The listing builds one solid part. Answer for the finished solid, in the listing's coordinates (mm). Face numbers are marked on the shaded views. A direction names the side the tool comes from. Round coordinates to 2 decimals unless told otherwise and drop trailing zeros. Write each loop counter-clockwise with the first axis right and the second up, starting at its lowest first coordinate (ties: lowest second). Pieces come first, ordered by that corner, then holes. Notation, with made-up numbers: (78, 7.25) - (97, 7.25) arc R17 ccw to (97, 28.25) - close; hole circle Ø4 at (-35.75, -33.75). An arc over 180 degrees is marked (long way). Return JSON: item names as keys, results as strings. Group by question number.
from build123d import *

# Parameters (mm, degrees)
BOSS_EXTRUDE1_DEPTH     = 110
BOSS_EXTRUDE2_START     = -105.9
BOSS_EXTRUDE2_DEPTH     = 211.8
CUT_EXTRUDE1_REACH      = 226.526
SKETCH3_R               = 3.175
F_1_4_CLEARANCE_HOLE1_D = 6.7564


with BuildPart() as part:
    # Sketch1 → Boss-Extrude1 (new body)
    with BuildSketch(Plane(origin=(0, 0, 0), x_dir=(1, 0, 0), z_dir=(0, 1, 0))):
        with BuildLine():
            Line((-14.05, 19.05), (14.05, 19.05))
            ThreePointArc((14.05, 19.05), (17.585533906, 17.585533906), (19.05, 14.05))
            Line((19.05, 14.05), (19.05, -14.05))
            ThreePointArc((19.05, -14.05), (17.585533906, -17.585533906), (14.05, -19.05))
            Line((14.05, -19.05), (-14.05, -19.05))
            ThreePointArc((-14.05, -19.05), (-17.585533906, -17.585533906), (-19.05, -14.05))
            Line((-19.05, -14.05), (-19.05, 14.05))
            ThreePointArc((-19.05, 14.05), (-17.585533906, 17.585533906), (-14.05, 19.05))
        make_face()
        with BuildLine():
            Line((-15.875, 14.05), (-15.875, -14.05))
            ThreePointArc((-15.875, -14.05), (-15.340469876, -15.340469876), (-14.05, -15.875))
            Line((-14.05, -15.875), (14.05, -15.875))
            ThreePointArc((14.05, -15.875), (15.340469876, -15.340469876), (15.875, -14.05))
            Line((15.875, -14.05), (15.875, 14.05))
            ThreePointArc((15.875, 14.05), (15.340469876, 15.340469876), (14.05, 15.875))
            Line((14.05, 15.875), (-14.05, 15.875))
            ThreePointArc((-14.05, 15.875), (-15.340469876, 15.340469876), (-15.875, 14.05))
        make_face(mode=Mode.SUBTRACT)
    extrude(amount=BOSS_EXTRUDE1_DEPTH)


with BuildPart() as body_2:
    # Mirror2: mirrored copy
    add(part.part.mirror(Plane(origin=(86.85, 0, 0), x_dir=(0, 0, 1), z_dir=(1, 0, 0))))


with BuildPart() as part_1:
    add(part.part)

    add(body_2.part)  # Boss-Extrude2 merges body 2
    # Sketch2 → Boss-Extrude2 (add)
    with BuildSketch(Plane(origin=(86.85, 0, 0), x_dir=(0, 0, -1), z_dir=(1, 0, 0)).offset(BOSS_EXTRUDE2_START)):
        with BuildLine():
            Line((-29.05, 148.1), (-0.95, 148.1))
            ThreePointArc((-0.95, 148.1), (2.585533906, 146.635533906), (4.05, 143.1))
            Line((4.05, 143.1), (4.05, 115))
            ThreePointArc((4.05, 115), (2.585533906, 111.464466094), (-0.95, 110))
            Line((-0.95, 110), (-29.05, 110))
            ThreePointArc((-29.05, 110), (-32.585533906, 111.464466094), (-34.05, 115))
            Line((-34.05, 115), (-34.05, 143.1))
            ThreePointArc((-34.05, 143.1), (-32.585533906, 146.635533906), (-29.05, 148.1))
        make_face()
        with BuildLine():
            Line((-30.875, 143.1), (-30.875, 115))
            ThreePointArc((-30.875, 115), (-30.340469876, 113.709530124), (-29.05, 113.175))
            Line((-29.05, 113.175), (-0.95, 113.175))
            ThreePointArc((-0.95, 113.175), (0.340469876, 113.709530124), (0.875, 115))
            Line((0.875, 115), (0.875, 143.1))
            ThreePointArc((0.875, 143.1), (0.340469876, 144.390469876), (-0.95, 144.925))
            Line((-0.95, 144.925), (-29.05, 144.925))
            ThreePointArc((-29.05, 144.925), (-30.340469876, 144.390469876), (-30.875, 143.1))
        make_face(mode=Mode.SUBTRACT)
    extrude(amount=BOSS_EXTRUDE2_DEPTH)

    # Cut-Extrude1: up to this face of the body (flat: up to its plane)
    cut_extrude1_end = Plane(part_1.part.faces().sort_by_distance((86.85, 148.1, 15))[0])
    # Sketch3 → Cut-Extrude1 (cut, up to the picked face)
    with BuildSketch(Plane.XZ.offset(-110), mode=Mode.PRIVATE) as cut_extrude1_sk1:
        with Locations(Location((86.8, 23.050000029, 0), (0, 0, 270))):
            Circle(SKETCH3_R)
    cut_extrude1_tool1 = split(extrude(cut_extrude1_sk1.sketch, amount=-CUT_EXTRUDE1_REACH, mode=Mode.PRIVATE), bisect_by=cut_extrude1_end, keep=Keep.BOTH, mode=Mode.PRIVATE)
    add(cut_extrude1_tool1.solids().sort_by(Axis((86.8, 110, 23.05), (0, 1, 0)))[0], mode=Mode.SUBTRACT)

    # 1/4 Clearance Hole1 (through all)
    with Locations(Plane.ZY.offset(19.05)):
        with Locations((-6.35, 15.24), (6.35, 21.59)):
            Hole(F_1_4_CLEARANCE_HOLE1_D / 2)


solid = part_1.part
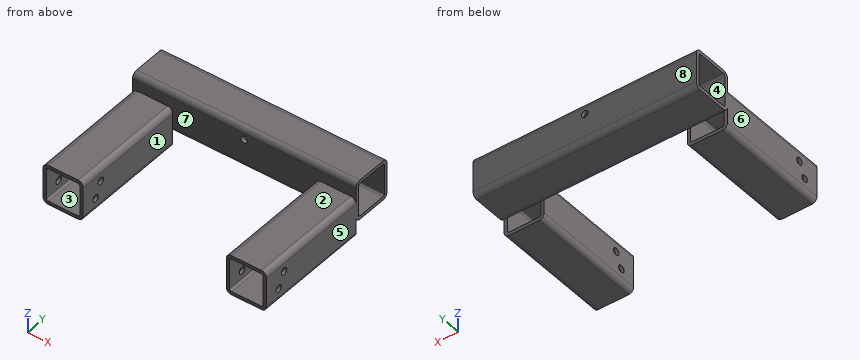
(1) Flat-ended cylindrical pins translate along their axes: pin 1 (14 mm diameter, centred on x = 167, y = 32, fed in from +Z); pin 2 (22.5 mm diameter, centred on x = 138, z = 12, fed in from -Y); pin 3 (2 mm diameter, centred on y = 18, z = 18.5, fed in from +X). Find the tip coordinate at first contact, or state that the pin passes through.
(2) Find section B-B (y = 123). Write down the section's boundary in (x, z) (3 decimals), plus the area to 3 significant figures.
(3) Find section A-A (y = 87). State how many separate pieces and enclosed holes the cut face has, plus the area to 3 significant figures.
(4) Consider line 1 (X direction, y = 47.5, z = 7) (3 decimals); line 2 (Y direction, x = 16.65, z = -6.35). Determine where each line is inside the solid, lowest interval first.
(5) Find section C-C (x = 86.8). Write down the section's boundary in (y, z) (3 decimals), plus the area to 3 significant figures.
(6) Determine the mould class of the marked faces 6, 7 and 8 for opening direction X: +X half, -X half, draft (parallel to the pull), parting line (faces both ways), or undercut.
(7) For the marked faces 1, 2, 3, 4 and 5, determine the directions among +Z, -Z, +X, -X, +Y, -Y from which every point of the face is accessible in a straight line to the end or side of a thin tool.
Check sheet entries:
{
 "1": {"pin 1": "stops at z = 19.05", "pin 2": "stops at y = 110", "pin 3": "stops at x = 191.37"},
 "2": {"outline": "(-19.05, -4.05) - (192.75, -4.05) - (192.75, -0.875) - (-19.05, -0.875) - close; (-19.05, 30.875) - (192.75, 30.875) - (192.75, 34.05) - (-19.05, 34.05) - close", "area": "1,340 mm^2"},
 "3": {"separate pieces": "2", "enclosed holes": "2", "area": "850 mm^2"},
 "4": {"line 1": "x = -19.05 to -15.875, 15.875 to 19.05, 154.65 to 157.825, 189.575 to 192.75", "line 2": "y = 0 to 11.86, 18.62 to 110"},
 "5": {"outline": "(110, 0.95) arc R5 ccw to (115, -4.05) - (143.1, -4.05) arc R5 ccw to (148.1, 0.95) - (148.1, 19.875) - (144.925, 19.875) - (144.925, 0.95) arc R1.825 cw to (143.1, -0.875) - (115, -0.875) arc R1.825 cw to (113.175, 0.95) - (113.175, 19.875) - (110, 19.875) - close; (110, 26.225) - (113.175, 26.225) - (113.175, 29.05) arc R1.825 cw to (115, 30.875) - (143.1, 30.875) arc R1.825 cw to (144.925, 29.05) - (144.925, 26.225) - (148.1, 26.225) - (148.1, 29.05) arc R5 ccw to (143.1, 34.05) - (115, 34.05) arc R5 ccw to (110, 29.05) - close", "area": "385 mm^2"},
 "6": {"face 6": "-X half", "face 7": "undercut", "face 8": "draft"},
 "7": {"face 1": "+Z, -Z, -Y", "face 2": "+Z, +X, -X, -Y", "face 3": "+Y, -Y", "face 4": "+X, -X", "face 5": "+Z, -Z, +X, +Y, -Y"}
}
